Geometry: final body of the model. Coordinates: model frame, mm. Face numbers are marked on the shaded views. A direction names the side the tool comes from. Coordinates: 2 decimals unless noted, no trailing zeros. Loops run counter-clockwise (first coordinate to the right, second up) from the corner with the lowest first, then second, coordinate; pieces in that order, holes last. Notation, with made-up numbers: (64.25, 58) - (88.25, 58) arc R17 ccw to (88.25, 85) - close; hole circle Ø7 at (80.25, 10). An arc over 180 degrees is marked (long way). Put each result on its own line as item: value. Start each with the question number.
1) Draft query along Z for the marked faces 5, 6 and 7. Return one class per face: +Z half, -Z half, draft (parallel to the pull), parting line (faces both ways), or undercut.
2) Material intervals for line 1 along X through (y, z) = (0, 7.9) (3 decimals); line 2 along X through (y, z) = (0, 6.2) (3 decimals); line 3 along Z through (x, y) = (18.5, 4.5) (3 decimals), sorted ascending. Write a range as from..to.
3) Section B-B on z = -3.5. Output: boundary loops of the cut face in (x, y) (3 decimals), and give its area (3 significant figures).
4) Reachability of the marked faces 1, 2, 3 and 4 from +Z, -Z, +X, -X, +Y, -Y: full face, straight path, thin tool, end or side. Return the list, or none.
5) Contact query for flat-ended pins moving along their axis: pin 1 Ø2 at (y, z) = (-1, -6.5) entering from -X (3 decimals); pin 2 Ø2.5 at (y, z) = (1.5, 7.5) entering from +X; pin 3 Ø1 at (x, y) = (6.5, -3) entering from -Z; pin 4 Ø4 at (y, z) = (7.5, 7.5) entering from -X. Output: stop coordinate, or through.
6) Section D-D on z = -6.5. Count the separate pieces of the cut face and the enclosed holes in it, and give its area (3 significant figures).
7) Section C-C on x = 24.5. Output: boundary loops of the cut face in (y, z) (3 decimals), and give its area (3 significant figures).
8) Section A-A on x = -4. Output: boundary loops of the cut face in (y, z) (3 decimals).
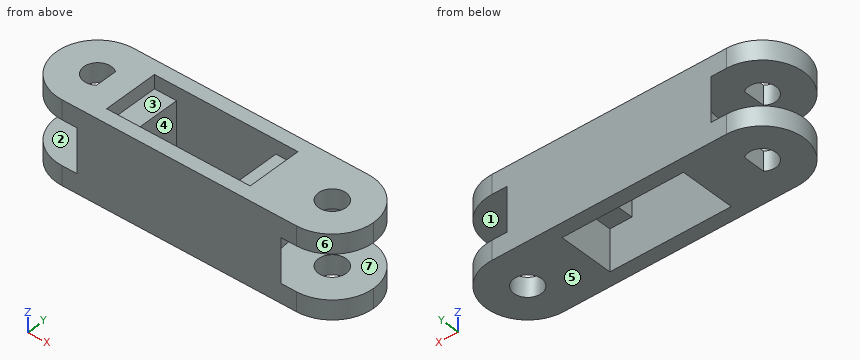
```python
from build123d import *

# Parameters (mm, degrees)
SKETCH1_W               = 63.5
SKETCH1_H               = 19.05
BOSS_EXTRUDE1_DEPTH     = 9.525
FILLET1_R               = 9.525
CUT_EXTRUDE1_DEPTH      = 39.232062788
CUT_EXTRUDE1_DEPTH_BACK = 39.232062788
SKETCH2_R               = 3.175
CUT_EXTRUDE2_DEPTH      = 39.232062788
CUT_EXTRUDE2_DEPTH_BACK = 3.175
SKETCH3_W               = 33.02
SKETCH3_H               = 12.7
SKETCH6_W               = 22.86
SKETCH6_H               = 12.7
CUT_EXTRUDE4_DEPTH      = 39.232062788
SKETCH7_W               = 5.08
SKETCH7_H               = 12.7
CUT_EXTRUDE5_DEPTH      = 9.525
BOSS_EXTRUDE2_DEPTH     = 19.05
CUT_EXTRUDE6_DEPTH      = 47.446245812
SKETCH4_R               = 10.16
CUT_EXTRUDE3_DEPTH      = 5.08


with BuildPart() as part:
    # Sketch1 → Boss-Extrude1 (new, symmetric)
    with BuildSketch(Plane.XY):
        Rectangle(SKETCH1_W, SKETCH1_H)
    extrude(amount=BOSS_EXTRUDE1_DEPTH, both=True)

    # Fillet1
    fillet1_edges = [part.edges().sort_by_distance(p)[0] for p in [
        (31.75, -9.525, 0),
        (31.75, 9.525, 0),
    ]]
    fillet(fillet1_edges, radius=FILLET1_R - 0.0001)  # a hair under: the kernel refuses the full size

    # Sketch2 → Cut-Extrude1 (cut, two sides: drawn at the far end of the back side and taken through both)
    with BuildSketch(Plane.XY.offset(9.525).offset(-CUT_EXTRUDE1_DEPTH_BACK)):
        with Locations((22.225, 0)):
            Circle(SKETCH2_R)
    extrude(amount=CUT_EXTRUDE1_DEPTH + CUT_EXTRUDE1_DEPTH_BACK, mode=Mode.SUBTRACT)

    # Sketch3 → Cut-Extrude2 (cut, two sides: drawn at the far end of the back side and taken through both)
    with BuildSketch(Plane.XY.offset(9.525).offset(-CUT_EXTRUDE2_DEPTH_BACK)):
        with Locations((-7.691525386, 0)):
            Rectangle(SKETCH3_W, SKETCH3_H)
    extrude(amount=CUT_EXTRUDE2_DEPTH + CUT_EXTRUDE2_DEPTH_BACK, mode=Mode.SUBTRACT)

    # Sketch6 → Cut-Extrude4 (cut, through all)
    with BuildSketch(Plane(origin=(0, 0, -9.525), x_dir=(-1, 0, 0), z_dir=(0, 0, -1))):
        with Locations((7.691525386, 0)):
            Rectangle(SKETCH6_W, SKETCH6_H)
    extrude(amount=-CUT_EXTRUDE4_DEPTH, mode=Mode.SUBTRACT)

    # Sketch7 → Cut-Extrude5 (cut)
    with BuildSketch(Plane(origin=(0, 0, -9.525), x_dir=(-1, 0, 0), z_dir=(0, 0, -1))):
        with Locations((-6.278474614, 0)):
            Rectangle(SKETCH7_W, SKETCH7_H)
    extrude(amount=-CUT_EXTRUDE5_DEPTH, mode=Mode.SUBTRACT)

    # Sketch8 → Boss-Extrude2 (add)
    with BuildSketch(Plane.XY.offset(9.525)):
        with BuildLine():
            Line((-31.75, 9.525), (-31.75, -9.525))
            ThreePointArc((-31.75, -9.525), (-41.275, 0), (-31.75, 9.525))
        make_face()
    extrude(amount=-BOSS_EXTRUDE2_DEPTH)

    # Sketch9 → Cut-Extrude6 (cut, through all)
    with BuildSketch(Plane.XY.offset(9.525)):
        with BuildLine():
            Line((-29.845, 2.54), (-29.845, -2.54))
            ThreePointArc((-29.845, -2.54), (-34.925, 0), (-29.845, 2.54))
        make_face()
    extrude(amount=-CUT_EXTRUDE6_DEPTH, mode=Mode.SUBTRACT)

    # Sketch4 → Cut-Extrude3 (cut, symmetric)
    with BuildSketch(Plane.XY):
        with Locations((22.225, 0)):
            Circle(SKETCH4_R)
        with Locations((-31.75, 0)):
            Circle(SKETCH4_R)
    extrude(amount=CUT_EXTRUDE3_DEPTH, both=True, mode=Mode.SUBTRACT)


solid = part.part
```
Answer block:
1. face 5: -Z half
1. face 6: draft
1. face 7: undercut
2. line 1: x = -41.275..-34.925, -29.845..-24.202, 8.818..19.05, 25.4..31.75
2. line 2: x = -41.275..-34.925, -29.845..-19.122, 3.738..19.05, 25.4..31.75
2. line 3: z = -9.525..-5.08, 5.08..9.525
3. outline: (-28.214, -9.525) - (18.689, -9.525) arc R10.16 cw to (18.689, 9.525) - (-28.214, 9.525) arc R10.16 cw to start; hole (-19.122, -6.35) - (8.818, -6.35) - (8.818, 6.35) - (-19.122, 6.35) - close
3. area: 355 mm²
4. face 1: +X
4. face 2: -X
4. face 3: +Z
4. face 4: +Z, -Z
5. pin 1: stops at x = -41.275
5. pin 2: stops at x = 31.75
5. pin 3: stops at z = 0
5. pin 4: stops at x = -39.53
6. separate pieces: 1
6. enclosed holes: 3
6. area: 900 mm²
7. outline: (-9.249, -9.525) - (-2.215, -9.525) - (-2.215, -5.08) - (-9.249, -5.08) - close; (-9.249, 5.08) - (-2.215, 5.08) - (-2.215, 9.525) - (-9.249, 9.525) - close; (2.215, -9.525) - (9.249, -9.525) - (9.249, -5.08) - (2.215, -5.08) - close; (2.215, 5.08) - (9.249, 5.08) - (9.249, 9.525) - (2.215, 9.525) - close
7. area: 125 mm²
8. outline: (-9.525, -9.525) - (-6.35, -9.525) - (-6.35, 9.525) - (-9.525, 9.525) - close; (6.35, -9.525) - (9.525, -9.525) - (9.525, 9.525) - (6.35, 9.525) - close
